Autodesk Inventor part; units mm, degrees
ref_plane "YZ Plane" through (0, 0, 0) normal (1, 0, 0) x (0, 1, 0)
ref_plane "XZ Plane" through (0, 0, 0) normal (0, 1, 0) x (-1, 0, 0)
ref_plane "XY Plane" through (0, 0, 0) normal (0, 0, 1) x (1, 0, 0)
sketch "Sketch1" plane through (0, 0, 0) normal (0, 1, 0) x (-1, 0, 0)
  line L0 (15, -35) -> (-15, -35)
  line L1 (-15, -35) -> (-15, 35)
  line L2 (-15, 35) -> (15, 35)
  line L3 (15, 35) -> (15, -35)
  line L4 (15, -35) -> (-15, 35) construction
  line L5 (-15, -35) -> (15, 35) construction
  point P0 (0, 0)
  dimension "d0" = 30
  dimension "d1" = 70
extrude "Extrusion1" add sketch "Sketch1" along normal blind 30
sketch "Sketch2" plane through (15, 0, 35) normal (1, 0, 0) x (0, 0, -1)
  circle A0 centre (35, 15.1375) radius 14.909
  line L0 (0, 0) -> (0, 30)
  line L1 (0, 8.8455) -> (70, 8.8455)
  line L2 (0, 30) -> (70, 30)
  line L3 (0, 0) -> (70, 0)
  line L4 (70, 0) -> (70, 30)
  point P0 (35, 0)
  point P1 (36.1767, 30)
  point P2 (21.4837, 8.8455)
  point P3 (33.8233, 30)
  point P4 (48.5163, 8.8455)
extrude "Extrusion2" cut sketch "Sketch2" against normal blind 30 contours A0 L2 L4 L1 | A0 L1 L0 L2
sketch "Sketch3" plane through (-15, 0, 35) normal (0, 0, 1) x (1, 0, 0)
  circle A0 centre (15, 19.3194) radius 10.5597
  line L0 (0, 30) -> (0, 8.8455)
  line L1 (0, 30) -> (30, 30)
  line L2 (30, 8.8455) -> (30, 30)
  line L3 (30, 8.8455) -> (0, 8.8455)
  point P0 (15, 0)
  point P1 (13.6563, 8.8455)
  point P2 (16.3437, 8.8455)
extrude "Extrusion3" cut sketch "Sketch3" against normal blind 77 contours A0 L3 L0 L1 L2
sketch "Sketch5" plane through (15, 8.8455, 35) normal (0, 1, 0) x (1, 0, 0)
  line L0 (-30, 0) -> (0, 0)
  line L1 (-30, 70) -> (-30, 0)
  line L2 (0, 0) -> (-30, 0)
  line L3 (-30, 0) -> (-30, 70)
  line L4 (-30, 70) -> (0, 70)
  line L5 (0, 70) -> (0, 0)
  point P0 (-15, 35)
extrude "Extrusion5" cut sketch "Sketch5" against normal up to surface (8.8455 mm away)
sketch "Sketch6" plane through (15, 8.8455, 35) normal (0, -1, 0) x (1, 0, 0)
  line L0 (-13.6563, -48.5163) -> (-16.3437, -48.5163)
  line L1 (-15, -48.5163) -> (-15, -21.5593) construction
  line L2 (-13.6563, -21.4837) -> (-13.6563, -48.5163)
  line L3 (-13.6563, -35) -> (-16.3437, -35) construction
  point P0 (-15, -35)
  point P1 (-15, -35)
properties part number "ball transfer unit" material "Stainless Steel"
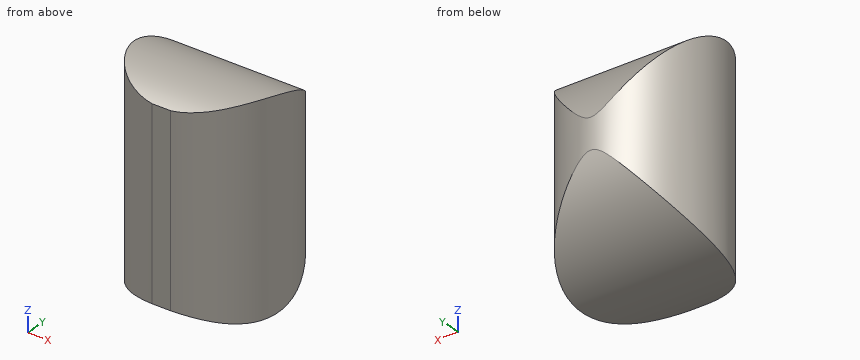
Geometry check sheet. Reference: the model listing, model coordinates, mm. Give positions to 0.01 mm unless a question says otherwise; leave off trailing zeros. Loops run counter-clockwise (first coordinate to the right, second up) from the corner with the lowest first, then second, coordinate; pieces in that order, holes last. Notation, with made-up numbers: M 28.25,55.25 L 60.25,55.25 A26 cw 60.25,74.25 Z; hole C 28,87 d7. An arc over 180 degrees is marked long. Write item = value, one per line. Start each with the question number.
1. Thickness scan on probe 1 along Z at (x, y) = (-4, 15); probe 2 along X at (y, z) = (19.5, -12); probe 3 along X at (y, z) = (21, 9.5). Record the ranges inside material, lowest first.
2. Section check B-B, the plane y = 25.75. Enter the section's corners in (x, z).
3. Section check A-A, the plane x = 0. Enter the section's corners in (y, z), plus the area to 3 significant figures.
4. Go/stop test with flat-tipped pins: P1, Ø4, axis at y = 25.5, z = 9.5, coming from the +X side; P2, Ø1.5, axis at x = 3, y = 24.5, coming from the -Z side; P3, Ø3, axis at x = -5, z = 0, coming from the +Y side. Record where each tip stops, or that it passes through.
Values follow:
q1.probe_1 = -14.91 to 14.91
q1.probe_2 = -10.56 to 10.56
q1.probe_3 = -10.43 to 10.43
q2.outline = M -8.38,-10.47 L 8.38,-10.47 L 8.38,10.47 L -8.38,10.47 Z
q3.outline = M 8.85,-13.52 A14.91 ccw 29.88,-2.23 L 29.88,2.23 A14.91 ccw 8.85,13.52 Z
q3.area = 531 mm^2
q4.P1 = 9.7
q4.P2 = -12.17
q4.P3 = 29.28
